Here's the drawing with two shaded views (mm, measured from the low corner). I have some questions. A direction names the side the tool comes from. Coordinates: 2 decimals unless noted, no trailing zeros. Write each loop counter-clockwise with the first axis right and the second up, starting at its lowest first coordinate (ties: lowest second). Pieces come first, ordered by that corner, then holes.
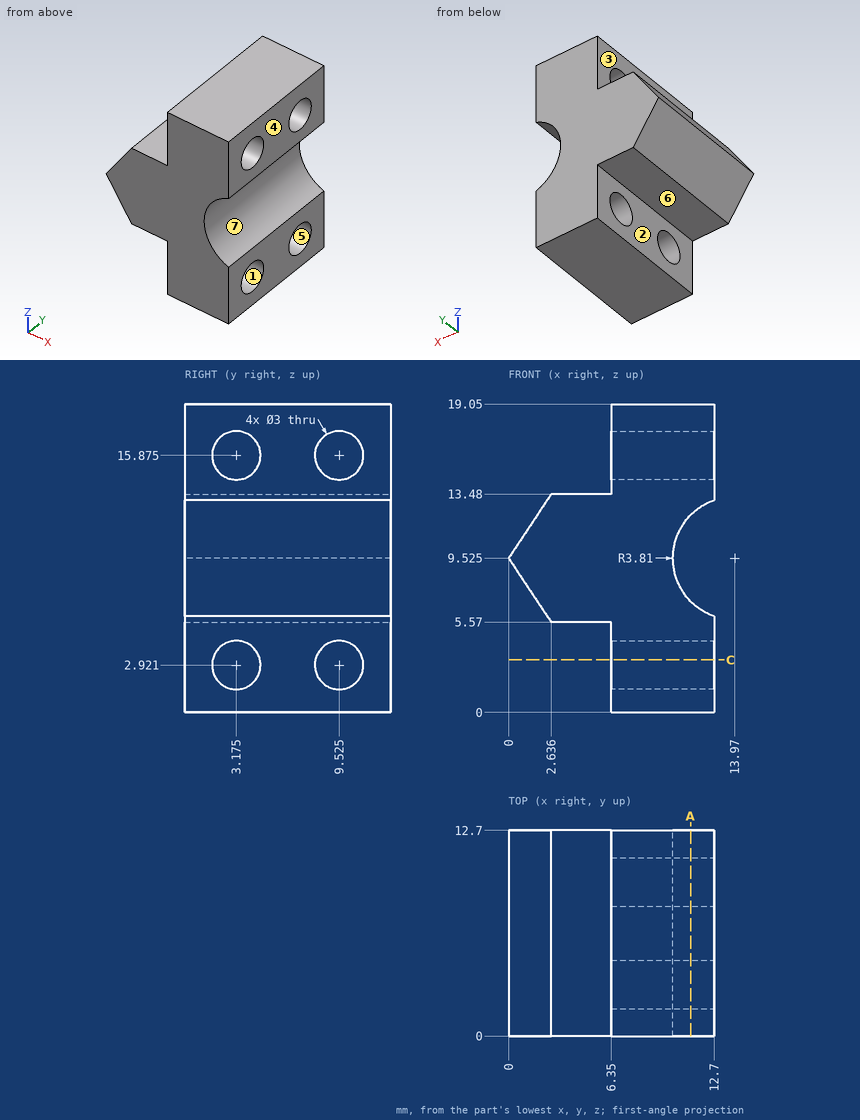
1. If we section it at C-C, the plane z = 3.25: List the corners of the cut face in (x, y) for me.
2. I'm going to push flat-ended pins straight in: P1, Ø5, axis at y = 2, z = 9.5, coming from the +X side; P2, Ø1.1, axis at x = 5, y = 4, coming from the -Z side; P3, Ø4.5, axis at y = 7, z = 17.5, coming from the -X side. Where does each tip first touch, or does it pass through?
3. If I drill on L1, parallel to Z at x = 5.75, y = 6.75; L2, parallel to X at y = 7.25, z = 14.5; L3, parallel to Z at x = 2, y = 5.25 (1 decimal), over which ranges is the centre line in solid material (lowest first)?
4. If we section it at A-A, the plane x = 11.25: Count the separate pieces of the cut face and the enclosed holes in it, plus the area to 3 significant figures.
5. We'd pull the mould along Z, two halves only. Please class the marked faces 4, 5, 6 and 7: released by +Z, released by -Z, zero draft, split by the parting line, or undercut.
6. Which directions (+Z, -Z, +X, -X, +Y, -Y) give clear straight access to the entire face, cutting with the end or side of a thin tool? Please do the marked faces 1, 2 and 3.
Answers:
1. outline: (6.35, 0) - (12.7, 0) - (12.7, 1.71) - (6.35, 1.71) - close; (6.35, 4.64) - (12.7, 4.64) - (12.7, 8.06) - (6.35, 8.06) - close; (6.35, 10.99) - (12.7, 10.99) - (12.7, 12.7) - (6.35, 12.7) - close
2. P1: stops at x = 11.12
2. P2: stops at z = 5.57
2. P3: stops at x = 6.35
3. L1: z = 5.57 to 13.48
3. L2: x = 6.35 to 12.7
3. L3: z = 6.5 to 12.5
4. separate pieces: 2
4. enclosed holes: 4
4. area: 146 mm2
5. face 4: zero draft
5. face 5: undercut
5. face 6: released by -Z
5. face 7: undercut
6. face 1: +X, -X
6. face 2: -Z, -X, +Y, -Y
6. face 3: +Z, -X, +Y, -Y
